Model file for the job. Use its own axes, mm. A direction names the side the tool comes from. Give positions to 0.01 mm unless a question says otherwise; leave off trailing zeros. Loops run counter-clockwise (first coordinate to the right, second up) from the corner with the lowest first, then second, coordinate; pieces in that order, holes last. Notation, with made-up numbers: M 13.5,-30 L 63.5,-30 A16 cw 63.5,-21 Z; hole C -10,-20.5 d1. An arc over 180 degrees is marked long. Use CSV: the item, a comma, the result in double quotes. Start each with the question number.
(1) Slice it at D-D on z = 27.5. List the corners of the cut face in (x, y), and give its area (3 significant figures).
(2) Two-plate mould, pull along Y, no slides. Class faces 4 (the face through (-6.827, 48.809, 6.261)), 5 (the face through (25.4, 10, 15)), 6 (the face through (0.559, 63.494, 6.261)): pulls with the +Y half, pulls with the -Y half, needs draft (parallel to the pull), parting line crosses it, or undercut.
(3) Slice it at C-C on y = 21. List the corners of the cut face in (x, z), and give its area (3 significant figures).
(4) Slice it at B-B on z = 4.5. List the corners of the cut face in (x, y).
(5) Flat gauge pins, fed straight in: P1, Ø8, axis at x = -18.5, y = 26, coming from the +Z side; P2, Ø10, axis at y = 5.5, z = 32, coming from the -X side; P3, Ø10, axis at x = -16, y = 8, coming from the +Z side; P4, Ø12, axis at x = 8, z = 23.5, coming from the +Y side. Where does each tip first touch, or does it go through?
(6) Tool access for faces 1 (the face through (0, 0, 19)), 2 (the face through (-19, 6, 25.4)), 3 (the face through (0, 12.7, 25)): list every direction of +Z, -Z, +X, -X, +Y, -Y with a clear straight run to the whole face (end or side of a thin tool).
(7) Wall check: line 1 along Y through (x, z) = (0, 8); line 2 along X through (y, z) = (38, 7); line 3 along Z through (x, y) = (8.5, 59.5). Give the ranges that are in metal, low to high. Write a range as from..to.
(8) Slice it at A-A on x = 0. List the corners of the cut face in (y, z), and give its area (3 significant figures).
```python
from build123d import *

# Parameters (mm, degrees)
F1_DEPTH = 12.7
F2_W     = 38.1
F2_H     = 12.7
F2_W_2   = 12.7
F3_DEPTH = 25.4
F4_W     = 12.7
F4_H     = 12.7
F5_DEPTH = 12.7


with BuildPart() as f1:
    # F0 (on Top) → F1 (new body)
    with BuildSketch(Plane.XY):
        with BuildLine():
            Line((-25.4, 38.1), (-25.4, 0))
            Line((-25.4, 0), (25.4, 0))
            Line((25.4, 0), (25.4, 38.1))
            Line((25.4, 38.1), (12.7, 38.1))
            ThreePointArc((12.7, 38.1), (0, 25.4), (-12.7, 38.1))
            Line((-12.7, 38.1), (-25.4, 38.1))
        make_face()
        with BuildLine():
            ThreePointArc((25.4, 38.1), (0, 63.5), (-25.4, 38.1))
            Line((-25.4, 38.1), (-12.7, 38.1))
            ThreePointArc((-12.7, 38.1), (0, 50.8), (12.7, 38.1))
            Line((12.7, 38.1), (25.4, 38.1))
        make_face()
    extrude(amount=F1_DEPTH)

    # F2 (on face) → F3 (join)
    with BuildSketch(Plane.XY.offset(12.7)):
        with Locations((6.35, 6.35)):
            Rectangle(F2_W, F2_H)
        with Locations((-19.05, 6.35)):
            Rectangle(F2_W_2, F2_H)
    extrude(amount=F3_DEPTH)

    # F4 (on face) → F5 (cut)
    with BuildSketch(Plane.XY.offset(38.1)):
        with Locations((-19.05, 6.35)):
            Rectangle(F4_W, F4_H)
    extrude(amount=-F5_DEPTH, mode=Mode.SUBTRACT)


solid = f1.part
```
Reply:
1,outline,"M -12.7,0 L 25.4,0 L 25.4,12.7 L -12.7,12.7 Z"
1,area,"484 mm^2"
2,face 4,"undercut"
2,face 5,"needs draft"
2,face 6,"pulls with the +Y half"
3,outline,"M -25.4,0 L 25.4,0 L 25.4,12.7 L -25.4,12.7 Z"
3,area,"645 mm^2"
4,outline,"M -25.4,0 L 25.4,0 L 25.4,38.1 A25.4 ccw -25.4,38.1 Z; hole C 0,38.1 d25.4"
5,P1,"stops at z = 12.7"
5,P2,"stops at x = -12.7"
5,P3,"stops at z = 38.1"
5,P4,"stops at y = 12.7"
6,face 1,"+Z, -Z, +X, -X, -Y"
6,face 2,"+Z, -X, +Y, -Y"
6,face 3,"+Z, +X, -X, +Y"
7,line 1,"y = 0..25.4, 50.8..63.5"
7,line 2,"x = -25.4..-12.7, 12.7..25.4"
7,line 3,"z = 0..12.7"
8,outline,"M 0,0 L 25.4,0 L 25.4,12.7 L 12.7,12.7 L 12.7,38.1 L 0,38.1 Z; M 50.8,0 L 63.5,0 L 63.5,12.7 L 50.8,12.7 Z"
8,area,"806 mm^2"
